For this review, take the finished solid that the model builds, in its own axes (mm). Round coordinates to 2 decimals unless told otherwise and drop trailing zeros. Loops run counter-clockwise (first coordinate to the right, second up) from the corner with the lowest first, then second, coordinate; pieces in that order, holes last. Notation, with made-up numbers: (20.5, -28) -> (73.5, -28) arc R19 cw to (73.5, -19) -> close; hole circle Ø3 at (9, 12.5). An arc over 180 degrees is marked (long way). Use one line per item in the form item = value. Start each with the question number.
from build123d import *

# Parameters (mm, degrees)
SKETCH_1_R      = 18
EXTRUDE_1_DEPTH = 10
SKETCH_2_R      = 1
EXTRUDE_2_DEPTH = 200
EXTRUDE_START   = 10
SKETCH_3_R      = 18
EXTRUDE_3_DEPTH = 10


with BuildPart() as part:
    # 草图1 → 凸台-拉伸1 (new body)
    with BuildSketch(Plane(origin=(0, 0, 0), x_dir=(1, 0, 0), z_dir=(0, 1, 0))):
        with Locations(Location((0, 0, 0), (0, 0, 270))):
            Circle(SKETCH_1_R)
    extrude(amount=EXTRUDE_1_DEPTH)

    # 草图2 → 凸台-拉伸2 (add)
    with BuildSketch(Plane(origin=(0, 0, 0), x_dir=(-1, 0, 0), z_dir=(0, -1, 0))):
        with Locations(Location((0, 0, 0), (0, 0, 270))):
            Circle(SKETCH_2_R)
    extrude(amount=EXTRUDE_2_DEPTH)

    # 草图3 → 凸台-拉伸3 (add)
    with BuildSketch(Plane(origin=(0, -200, 0), x_dir=(-1, 0, 0), z_dir=(0, -1, 0)).offset(EXTRUDE_START)):
        with Locations(Location((0, 0, 0), (0, 0, 270))):
            Circle(SKETCH_3_R)
    extrude(amount=-EXTRUDE_3_DEPTH)


solid = part.part
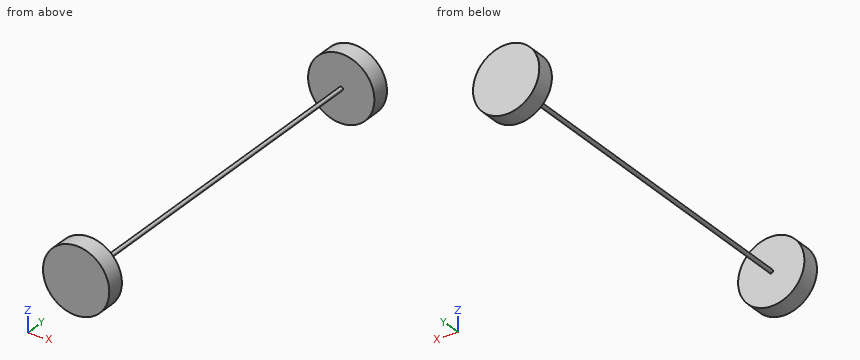
Item 1: Take a section at C-C on y = -26. Give the boundary of the cut face in (x, z), plus the area to 3 significant figures.
Item 2: Wall thickness on line 1 (Y direction, x = 15.5, z = -2): over which ranges is the line inside the solid? List them lowest first.
Item 3: Take a section at A-A on z = 13. Give the boundary of the cut face in (x, y), plus the area to 3 significant figures.
Item 4: For P1, Ø10, axis at x = -5.5, y = -107.5, coming from the +Z side; P2, Ø10, axis at y = -107, z = 10, coming from the +X side, all flat-tipped, find the tip position at first contact; note any pin that passes through.
Item 5: Take a section at B-B on x = -11.5. Give the boundary of the cut face in (y, z), plus the area to 3 significant figures.
Results:
q1.outline = circle Ø2 at (0, 0)
q1.area = 3.14 mm2
q2.line_1 = -210 to -200, 0 to 10
q3.outline = (-12.45, -210) -> (12.45, -210) -> (12.45, -200) -> (-12.45, -200) -> close; (-12.45, 0) -> (12.45, 0) -> (12.45, 10) -> (-12.45, 10) -> close
q3.area = 498 mm2
q4.P1 = 0.87
q4.P2 = through
q5.outline = (-210, -13.85) -> (-200, -13.85) -> (-200, 13.85) -> (-210, 13.85) -> close; (0, -13.85) -> (10, -13.85) -> (10, 13.85) -> (0, 13.85) -> close
q5.area = 554 mm2
